Autodesk Inventor part; units mm, degrees
ref_plane "YZ Plane" through (0, 0, 0) normal (1, 0, 0) x (0, 1, 0)
ref_plane "XZ Plane" through (0, 0, 0) normal (0, 1, 0) x (-1, 0, 0)
ref_plane "XY Plane" through (0, 0, 0) normal (0, 0, 1) x (1, 0, 0)
sketch "Sketch1" plane through (0, 0, 0) normal (0, 0, 1) x (1, 0, 0)
  line L0 (21.5871, 13.6345) -> (17.0871, 18.1345)
  line L1 (17.0871, 18.1345) -> (-16.7129, 18.1345)
  line L2 (-16.7129, 18.1345) -> (-21.2129, 13.6345)
  line L3 (-21.0966, 13.6345) -> (-21.0966, -20.1655)
  line L4 (21.4709, -20.1655) -> (21.4709, 13.6345)
  line L5 (21.4709, -20.1655) -> (17.0871, -24.4078)
  line L6 (-16.7129, -24.4078) -> (17.0871, -24.4078)
  line L7 (-16.7129, -24.4078) -> (-21.0966, -20.1655)
  line L8 (-24.7129, -28.1655) -> (-24.7129, 13.6345) construction
  line L9 (25.0871, -28.1655) -> (-24.7129, -28.1655) construction
  line L10 (25.0871, -28.1655) -> (25.0871, 13.6345) construction
  line L11 (17.0871, 21.6345) -> (-16.7129, 21.6345) construction
  line L12 (0.1871, -36.5255) -> (0.1871, 21.9945)
  line L13 (-21.0552, -20.0655) -> (-16.6129, -24.5078)
  line L14 (-16.6129, -24.5078) -> (-16.6129, -28.1655)
  line L15 (-16.6129, -28.1655) -> (16.9871, -28.1655)
  line L16 (16.9871, -28.1655) -> (16.9871, -24.5078)
  line L17 (16.9871, -24.5078) -> (21.4295, -20.0655)
  line L18 (25.0871, -20.0655) -> (21.4295, -20.0655)
  line L19 (25.0871, 13.5345) -> (25.0871, -20.0655)
  line L20 (21.4295, 13.5345) -> (25.0871, 13.5345)
  line L21 (21.4295, 13.5345) -> (16.9871, 17.9768)
  line L22 (16.9871, 17.9768) -> (16.9871, 21.6345)
  line L23 (16.9871, 21.6345) -> (-16.6129, 21.6345)
  line L24 (-16.6129, 21.6345) -> (-16.6129, 17.9768)
  line L25 (-16.6129, 17.9768) -> (-21.0552, 13.5345)
  line L26 (-24.7129, 13.5345) -> (-21.0552, 13.5345)
  line L27 (-24.7129, -20.0655) -> (-24.7129, 13.5345)
  line L28 (-21.0552, -20.0655) -> (-24.7129, -20.0655)
  circle A0 centre (0.1871, -3.2655) radius 12.5 construction
  circle A1 centre (0.1871, -3.2655) radius 16.9 construction
  circle A2 centre (0.1871, -3.2655) radius 7.5 construction
  line L29 (0.547, -12.2476) -> (0.8041, -10.7401)
  arc A3 (-10.8411, 9.29) -> (0.8041, -10.7401) centre (-0.9086, 1.6644) ccw
  arc A4 (-14.6035, 4.5126) -> (0.547, -12.2476) centre (-0.9086, 1.6644) ccw
  arc A5 (-5.1721, -19.094) -> (6.3518, 1.0061) centre (-3.5344, -6.6794) ccw
  arc A6 (0.8464, -19.9636) -> (7.786, 1.5372) centre (-3.5344, -6.6794) ccw
  line L30 (7.786, 1.5372) -> (6.3518, 1.0061)
  arc A7 (16.5746, 0.0075) -> (-6.5945, -0.0625) centre (5.0044, -4.7815) ccw
  arc A8 (14.3185, 5.6545) -> (-7.7715, 0.914) centre (5.0044, -4.7815) ccw
  line L31 (-7.7715, 0.914) -> (-6.5945, -0.0625)
  arc A9 (0.1871, -19.9766) -> (0.8464, -19.9636) centre (0.211, -4.4767) ccw
  arc A10 (-12.8462, 5.1239) -> (-13.1888, 4.5662) centre (0.1871, -3.2655) ccw
  arc A11 (-12.8462, 5.1239) -> (-13.1888, 4.5662) centre (0.1871, -3.2655) ccw
  arc A12 (14.3185, 5.6545) -> (-10.8411, 9.29) centre (0.1871, -3.2655) ccw construction
  arc A13 (14.3185, 5.6545) -> (-10.8411, 9.29) centre (0.1871, -3.2655) ccw
  arc A14 (-14.6035, 4.5126) -> (-5.1721, -19.094) centre (0.1871, -3.2655) ccw construction
  arc A15 (0.1871, -19.9766) -> (16.5746, 0.0075) centre (0.1871, -3.2655) ccw construction
  arc A16 (-14.6035, 4.5126) -> (-5.1721, -19.094) centre (0.1871, -3.2655) ccw
  arc A17 (0.1871, -19.9766) -> (16.5746, 0.0075) centre (0.1871, -3.2655) ccw
  circle A18 centre (0.1871, -3.2655) radius 20
  point P0 (14.2, -44.8454)
  point P1 (16.9871, 19.8057)
  dimension "d49" = 15
  dimension "d48" = 25
  dimension "d53" = 360
  dimension "d61" = 40
extrude "Extrusion1" add sketch "Sketch1" along normal blind 5 contours L22 L21 L20 L4 L18 L17 L6 L12 A18 L1 | L1 L12 L23 L22 | L12 A18 L6 L13 L28 L3 L26 L25 L24 L1 | L1 L24 L23 L12 | L20 L19 L18 L4 | L12 L15 L14 L13 L6 | L6 L17 L16 L15 L12 | L3 L28 L27 L26
sketch "Sketch3" plane through (0, 0, 5) normal (0, 0, 1) x (1, 0, 0)
  circle A0 centre (0.1871, -3.2655) radius 20
  circle A1 centre (0.1871, -3.2655) radius 7.5 construction
  arc A2 (-2.7759, 3.6244) -> (0.1871, -23.2655) centre (2.8116, -9.3681) ccw
  arc A3 (-3.7493, 5.3815) -> (-7.6417, -21.6695) centre (2.8116, -9.3681) ccw
  line L0 (-3.7493, 5.3815) -> (-2.7759, 3.6244)
  arc A4 (-7.6417, -21.6695) -> (0.1871, -23.2655) centre (0.1871, -3.2655) ccw
  point P0 (0, 0)
  dimension "d55" = 15
  dimension "d62" = 2
extrude "Extrusion3" add sketch "Sketch3" against normal up to surface (5 mm away) contours A3 L0 A2 A0 picked at (-8.119, 1.4619)
pattern_circular "Circular Pattern1" count 3 over 360 about axis through (0.1871, -3.2655, 0) along (0, 0, 1) of "Extrusion3"
sketch "Sketch4" plane through (-24.7129, -20.0655, 0) normal (-1, 0, 0) x (0, 0, 1)
  line L0 (0, 41.7) -> (5, 41.7)
  point P0 (0, 20.0655)
  point P1 (2.5, 16.75)
  dimension "d63" = 24.95
hole "Hole1" at (-24.7129, -3.3155, 2.5) direction (1, 0, 0) diameter 2.9 depth 5 tip angle 118
pattern_circular "Circular Pattern2" count 4 over 360 about axis through (0.1871, -3.2655, 0) along (0, 0, 1) of "Hole1"
sketch "Skizze5" plane through (0, 0, 5) normal (0, 0, 1) x (1, 0, 0)
  arc A0 (-17.1334, 6.7345) -> (-7.6417, -21.6695) centre (0.1871, -3.2655) ccw construction
  arc A1 (7.6355, -4.1444) -> (-17.1334, 6.7345) centre (-6.4101, -2.487) ccw construction
  line L0 (7.6355, -4.1444) -> (9.6439, -4.1799) construction
  arc A2 (9.6439, -4.1799) -> (-11.8368, 12.7165) centre (-6.4101, -2.487) ccw construction
  arc A3 (17.5076, 6.7345) -> (-11.8368, 12.7165) centre (0.1871, -3.2655) ccw construction
  arc A4 (-4.2982, -9.2765) -> (17.5076, 6.7345) centre (4.1599, 2.0586) ccw construction
  line L1 (-4.2982, -9.2765) -> (-5.3332, -10.9981) construction
  arc A5 (-5.3332, -10.9981) -> (20.0399, -0.8435) centre (4.1599, 2.0586) ccw construction
  arc A6 (0.1871, -23.2655) -> (20.0399, -0.8435) centre (0.1871, -3.2655) ccw construction
  arc A7 (-2.7759, 3.6244) -> (0.1871, -23.2655) centre (2.8116, -9.3681) ccw construction
  line L2 (-2.7759, 3.6244) -> (-3.7493, 5.3815) construction
  arc A8 (-3.7493, 5.3815) -> (-7.6417, -21.6695) centre (2.8116, -9.3681) ccw construction
  line L3 (-21.0552, -20.0655) -> (-16.6129, -24.5078)
  line L4 (-16.6129, -24.5078) -> (-16.6129, -28.1655)
  line L5 (-16.6129, -28.1655) -> (16.9871, -28.1655) construction
  line L6 (16.9871, -28.1655) -> (16.9871, -24.5078)
  line L7 (16.9871, -24.5078) -> (21.4295, -20.0655)
  line L8 (21.4295, -20.0655) -> (25.0871, -20.0655)
  line L9 (25.0871, -20.0655) -> (25.0871, 13.5345) construction
  line L10 (25.0871, 13.5345) -> (21.4295, 13.5345)
  line L11 (21.4295, 13.5345) -> (16.9871, 17.9768)
  line L12 (16.9871, 17.9768) -> (16.9871, 21.6345)
  line L13 (16.9871, 21.6345) -> (-16.6129, 21.6345) construction
  line L14 (-16.6129, 21.6345) -> (-16.6129, 17.9768)
  line L15 (-16.6129, 17.9768) -> (-21.0552, 13.5345)
  line L16 (-21.0552, 13.5345) -> (-24.7129, 13.5345)
  line L17 (-24.7129, 13.5345) -> (-24.7129, -20.0655) construction
  line L18 (-24.7129, -20.0655) -> (-21.0552, -20.0655)
  line L19 (-16.7129, 21.7345) -> (17.0871, 21.7345) construction
  line L20 (17.0871, 21.7345) -> (17.0871, 18.0183)
  line L21 (17.0871, 18.0183) -> (21.4709, 13.6345)
  line L22 (21.4709, 13.6345) -> (25.1871, 13.6345)
  line L23 (25.1871, 13.6345) -> (25.1871, -20.1655) construction
  line L24 (25.1871, -20.1655) -> (21.4709, -20.1655)
  line L25 (21.4709, -20.1655) -> (17.0871, -24.5493)
  line L26 (17.0871, -24.5493) -> (17.0871, -28.2655)
  line L27 (17.0871, -28.2655) -> (-16.7129, -28.2655) construction
  line L28 (-16.7129, -28.2655) -> (-16.7129, -24.5493)
  line L29 (-16.7129, -24.5493) -> (-21.0966, -20.1655)
  line L30 (-21.0966, -20.1655) -> (-24.8129, -20.1655)
  line L31 (-24.8129, -20.1655) -> (-24.8129, 13.6345) construction
  line L32 (-24.8129, 13.6345) -> (-21.0966, 13.6345)
  line L33 (-21.0966, 13.6345) -> (-16.7129, 18.0183)
  line L34 (-16.7129, 18.0183) -> (-16.7129, 21.7345)
  line L35 (-24.7129, 13.5345) -> (-24.7129, 13.6345)
  line L36 (-16.6129, 21.6345) -> (-16.7129, 21.6345)
  line L37 (16.9871, 21.6345) -> (17.0871, 21.6345)
  line L38 (25.0871, 13.5345) -> (25.0871, 13.6345)
  line L39 (25.0871, -20.0655) -> (25.0871, -20.1655)
  line L40 (16.9871, -28.1655) -> (17.0871, -28.1655)
  line L41 (-16.6129, -28.1655) -> (-16.7129, -28.1655)
  line L42 (-24.7129, -20.0655) -> (-24.7129, -20.1655)
  point P0 (0, 0)
  dimension "d74" = 0.1
extrude "IM_offset" add sketch "Skizze5" against normal up to surface (5 mm away)
properties part number "20_Cube_Insert_Laser_Holder_v2"
Geometry check sheet. Reference: the model listing, model coordinates, mm. A direction names the side the tool comes from. Round coordinates to 2 decimals unless told otherwise and drop trailing zeros. Loops run counter-clockwise (first coordinate to the right, second up) from the corner with the lowest first, then second, coordinate; pieces in that order, holes last. Notation, with made-up numbers: (85.25, 33.25) - (95.25, 33.25) arc R12 cw to (95.25, 55.25) - close; hole circle Ø8 at (6, 31). An arc over 180 degrees is marked (long way). Answer as CSV lines item,"result".
(1) Material ranges on line 1 along Y through (x, z) = (15.5, 4.3); line 2 along X through (y, z) = (-16.5, 4.7); line 3 along Y through (x, z) = (0, 0.65), recorded low to high.
Output values:
line 1,"y = -28.17 to -16.13, -9.43 to -6.39, 9.6 to 21.63"
line 2,"x = -24.71 to -14.81, -11.67 to -9.4, 15.18 to 25.09"
line 3,"y = -28.17 to -23.23, -13.54 to -11.46, 10.12 to 12.33, 16.73 to 21.63"
(2) Release check for a two-part mould opening along Y. For faces 5 (the face through (-0.493, 10.358, 2.535)), 6 (the face through (-23, -20.166, 3)), 7 (the face through (-6, 3, 0)), 8 (the face through (-22.2, -2.43, 1.35)) record: released by +Y, released by -Y, zero draft, split by the parting line, or undercut.
Output values:
face 5,"undercut"
face 6,"released by -Y"
face 7,"zero draft"
face 8,"undercut"
(3) Depth check by flat-ended pin: pin 1 Ø3 at (y, z) = (-27, 3) entering from -X; pin 2 Ø3 at (y, z) = (-27, 2) entering from +X; pin 3 Ø2.5 at (y, z) = (-3.32, 2.5) entering from -X; pin 4 Ø1.5 at (x, y) = (0, -16) entering from -Z. Enter the tip coordinate at first touch or a pass-through.
Output values:
pin 1,"stops at x = -16.71"
pin 2,"stops at x = 17.09"
pin 3,"stops at x = -12.6"
pin 4,"passes through"
(4) Cross-section at C-C, the plane y = -8. Enter the section's corners in (x, z).
Output values:
outline,"(-24.71, 0) - (-19.24, 0) - (-19.24, 5) - (-24.71, 5) - close; (-13.27, 0) - (-11.27, 0) - (-11.27, 5) - (-13.27, 5) - close; (14.1, 0) - (16.79, 0) - (16.79, 5) - (14.1, 5) - close; (19.62, 0) - (25.09, 0) - (25.09, 5) - (19.62, 5) - close"
(5) Cross-section at B-B, the plane x = 16.5. Enter the section's corners in (y, z), and give its area (3 significant figures).
Output values:
outline,"(-28.17, 0) - (-14.84, 0) - (-14.84, 5) - (-28.17, 5) - close; (-8.35, 0) - (-4.85, 0) - (-4.85, 5) - (-8.35, 5) - close; (8.31, 0) - (21.63, 0) - (21.63, 5) - (8.31, 5) - close"
area,"151 mm²"
(6) Set-up check for faces 1 (the face through (-23, 13.634, 3)), 2 (the face through (22.57, -4.1, 1.35)), 3 (the face through (17.087, 20, 3)), 4 (the face through (-4.823, -10.149, 2.535)): record each of +Z, -Z, +X, -X, +Y, -Y from which the full face is reachable in a straight line by a thin tool's end or side.
Output values:
face 1,"+Z, -Z, -X, +Y"
face 2,"+X"
face 3,"+Z, -Z, +X, +Y"
face 4,"+Z, -Z"
(7) Cross-section at A-A, the plane y = 10. Enter the section's corners in (x, z), and give its area (3 significant figures).
Output values:
outline,"(-24.71, 0) - (-13.05, 0) - (-13.05, 5) - (-24.71, 5) - close; (0.23, 0) - (3.82, 0) - (3.82, 5) - (0.23, 5) - close; (15.15, 0) - (25.09, 0) - (25.09, 5) - (15.15, 5) - close"
area,"126 mm²"
(8) Cross-section at D-D, the plane x = -9. Enter the section's corners in (y, z), and give its area (3 significant figures).
Output values:
outline,"(-28.17, 0) - (-21.03, 0) - (-21.03, 5) - (-28.17, 5) - close; (-20.37, 0) - (-17.15, 0) - (-17.15, 5) - (-20.37, 5) - close; (-1.59, 0) - (1.64, 0) - (1.64, 5) - (-1.59, 5) - close; (11.42, 0) - (13.45, 0) - (13.45, 5) - (11.42, 5) - close; (14.5, 0) - (21.63, 0) - (21.63, 5) - (14.5, 5) - close"
area,"114 mm²"
